The model under review builds one solid part; all positions refer to its coordinate system, in mm. Face numbers are marked on the shaded views. A direction names the side the tool comes from. Coordinates: 2 decimals unless noted, no trailing zeros. Write each loop counter-clockwise with the first axis right and the second up, starting at its lowest first coordinate (ties: lowest second). Pieces come first, ordered by that corner, then holes. Notation, with made-up numbers: (7, 76.5) -> (52, 76.5) arc R10 ccw to (52, 86.5) -> close; hole circle Ø6 at (-21, 38). An arc over 180 degrees is marked (long way). Write each question's results on one line, items separated by ' | '.
```python
from build123d import *

# Parameters (mm, degrees)
F0_R     = 3.556
F0_R_2   = 5.334
F1_DEPTH = 7.62


with BuildPart() as f1:
    # F0 (on Front) → F1 (new body)
    with BuildSketch(Plane.XZ):
        with BuildLine():
            ThreePointArc((-5.233176, 7.186513), (0, 8.89), (5.233176, 7.186513))
            Line((5.233176, 7.186513), (5.233176, 16.354866))
            ThreePointArc((5.233176, 16.354866), (0, 13.601582), (-5.233176, 16.354866))
            Line((-5.233176, 16.354866), (-5.233176, 7.186513))
        make_face()
        with BuildLine():
            ThreePointArc((-5.233176, 16.354866), (0, 13.601582), (5.233176, 16.354866))
            ThreePointArc((5.233176, 16.354866), (6.06437, 18.068522), (6.35, 19.951582))
            ThreePointArc((6.35, 19.951582), (-1.88306, 26.015952), (-5.233176, 16.354866))
        make_face()
        with Locations((0, 19.951582)):
            Circle(F0_R, mode=Mode.SUBTRACT)
        with BuildLine():
            ThreePointArc((-5.233176, 7.186513), (-4.031697, -7.923227), (8.89, 0))
            ThreePointArc((8.89, 0), (7.923227, 4.031697), (5.233176, 7.186513))
            ThreePointArc((5.233176, 7.186513), (0, 8.89), (-5.233176, 7.186513))
        make_face()
        Circle(F0_R_2, mode=Mode.SUBTRACT)
    extrude(amount=F1_DEPTH)


solid = f1.part
```
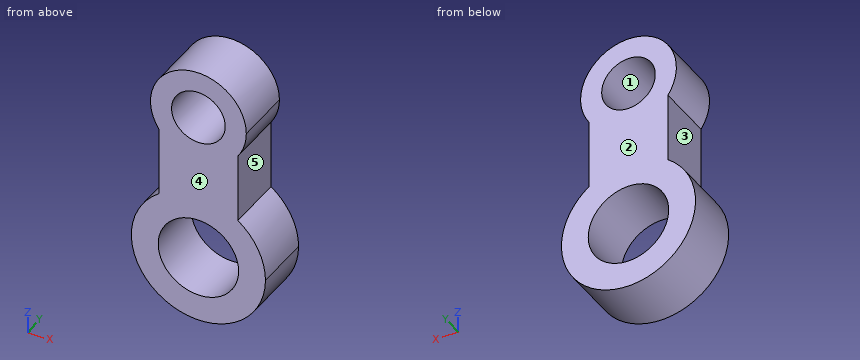
Q1. Clearance check with flat-ended pins moving along their axes: P1, Ø6.5, axis at x = 0, z = 0, coming from the +Y side; P2, Ø3, axis at y = -2, z = 20.5, coming from the -X side; P3, Ø3, axis at y = -2.5, z = 16, coming from the +X side; P4, Ø1, axis at y = -2.5, z = 7.5, coming from the -X side. State where each tip first meets the part, or that it passes through.
Solution:
P1: through | P2: x = -6.35 | P3: x = 5.86 | P4: x = -5.48
Q2. Add section B-B (y = -5.75). Write out the cut boundary in (x, z).
Solution:
outline: (-5.23, 7.19) arc R8.89 ccw (long way) to (8.89, 0) arc R8.89 ccw to (5.23, 7.19) -> (5.23, 16.35) arc R6.35 ccw (long way) to (-5.23, 16.35) -> close; hole circle Ø10.67 at (0, 0); hole circle Ø7.11 at (0, 19.95)
Q3. Add section C-C (z = 23). Write out the cut boundary in (x, y).
Solution:
outline: (-5.57, -7.62) -> (-1.83, -7.62) -> (-1.83, 0) -> (-5.57, 0) -> close; (1.83, -7.62) -> (5.57, -7.62) -> (5.57, 0) -> (1.83, 0) -> close
Q4. Machinability: for the marked faces 4 and 5, which of the approach directions +Z, -Z, +X, -X, +Y, -Y give a long, thin tool a straight path to every point of the face, cutting with its end or side? Answer none if there is none.
Solution:
face 4: +Z, -Z, +X, -X, -Y | face 5: +X, +Y, -Y
Q5. For line 1 (Z direction, x = 0, y = -5.5); line 2 (Z direction, x = 0.75, y = -2.5); line 3 (X direction, y = -5, z = -4.5), list the stretches that pass through material, from the lowest coordinate up. Write a range as from..to.
Solution:
line 1: -8.89..-5.33, 5.33..16.4, 23.51..26.3 | line 2: -8.86..-5.28, 5.28..16.48, 23.43..26.26 | line 3: -7.67..-2.86, 2.86..7.67
Q6. Draft analysis for pull direction X (two halves, no side actions). For the marked faces 1, 2 and 3, state which applies: pulls with the +X half, pulls with the -X half, needs draft (parallel to the pull), parting line crosses it, or undercut.
Solution:
face 1: undercut | face 2: needs draft | face 3: pulls with the -X half
Q7. Add section A-A (x = 0). Write out the cut boundary in (y, z), plus the area to 3 significant figures.
Solution:
outline: (-7.62, -8.89) -> (0, -8.89) -> (0, -5.33) -> (-7.62, -5.33) -> close; (-7.62, 5.33) -> (0, 5.33) -> (0, 16.4) -> (-7.62, 16.4) -> close; (-7.62, 23.51) -> (0, 23.51) -> (0, 26.3) -> (-7.62, 26.3) -> close | area: 133 mm²
Q8. Add section D-D (z = 19). Write out the cut boundary in (x, y), plus the area to 3 significant figures.
Solution:
outline: (-6.28, -7.62) -> (-3.43, -7.62) -> (-3.43, 0) -> (-6.28, 0) -> close; (3.43, -7.62) -> (6.28, -7.62) -> (6.28, 0) -> (3.43, 0) -> close | area: 43.5 mm²
